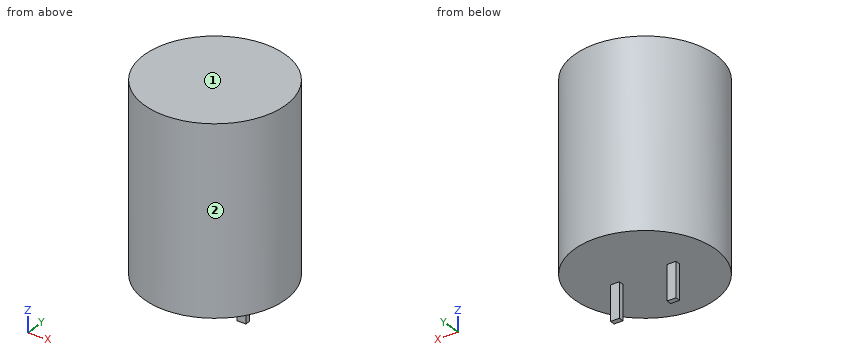
from build123d import *

# Parameters (mm, degrees)
SKETCH1_R           = 12.446
BOSS_EXTRUDE1_DEPTH = 32.512
SKETCH2_W           = 1.565145042
SKETCH2_H           = 0.889
BOSS_EXTRUDE2_DEPTH = 6.1


with BuildPart() as part:
    # Sketch1 → Boss-Extrude1 (new body)
    with BuildSketch(Plane.XY):
        Circle(SKETCH1_R)
    extrude(amount=BOSS_EXTRUDE1_DEPTH)

    # Sketch2 → Boss-Extrude2 (add)
    with BuildSketch(Plane.XY):
        with Locations((-5, 0)):
            Rectangle(SKETCH2_W, SKETCH2_H)
        with Locations((5, 0)):
            Rectangle(SKETCH2_W, SKETCH2_H)
    extrude(amount=-BOSS_EXTRUDE2_DEPTH)


solid = part.part
CAD build for the part. Positions are in the model's coordinates, mm. Face numbers are marked on the shaded views. Give positions to 0.01 mm unless a question says otherwise; leave off trailing zeros. Loops run counter-clockwise (first coordinate to the right, second up) from the corner with the lowest first, then second, coordinate; pieces in that order, holes last. Notation, with made-up numbers: M 61.5,31.5 L 89.5,31.5 A14 cw 89.5,45.5 Z; hole C -14,-17.5 d4. An arc over 180 degrees is marked long. One line per question, with ' | ' between items. Start each with the question number.
1. Saw through at C-C on z = 27. Give the cut face in (x, y).
2. Saw through at A-A on y = 0. Give the cut face in (x, z), plus the area to 3 significant figures.
3. Saw through at D-D on y = 10.75. Give the cut face in (x, z).
4. Two-plate mould, pull along X, no slides. Class the marked faces 1 and 2: pulls with the +X half, pulls with the -X half, needs draft (parallel to the pull), parting line crosses it, or undercut.
5. Probe L1, parallel to Z at x = -8.5, y = -5; L2, parallel to Y at x = 0, z = 21; L3, parallel to X at y = 6.5, z = 9. List the from-to ranges inside material, lowest first. Write a range as from..to.
6. Flat gauge pins, fed straight in: pin 1 (3 mm diameter, centred on x = -7.5, y = 8.5, fed in from -Z); pin 2 (0.8 mm diameter, centred on x = 5, z = -2, fed in from +Y); pin 3 (8 mm diameter, centred on x = 4.5, z = 1.5, fed in from -Y). Where does each tip first touch, or does it go through?
7. Saw through at B-B on x = 0. Give the cut face in (y, z).
Result sheet:
1) outline: C 0,0 d24.89
2) outline: M -12.45,0 L -5.78,0 L -5.78,-6.1 L -4.22,-6.1 L -4.22,0 L 4.22,0 L 4.22,-6.1 L 5.78,-6.1 L 5.78,0 L 12.45,0 L 12.45,32.51 L -12.45,32.51 Z | area: 828 mm^2
3) outline: M -6.27,0 L 6.27,0 L 6.27,32.51 L -6.27,32.51 Z
4) face 1: needs draft | face 2: parting line crosses it
5) L1: z = 0..32.51 | L2: y = -12.45..12.45 | L3: x = -10.61..10.61
6) pin 1: stops at z = 0 | pin 2: stops at y = 0.44 | pin 3: stops at y = -12.44
7) outline: M -12.45,0 L 12.45,0 L 12.45,32.51 L -12.45,32.51 Z
